```python
from build123d import *

# Parameters (mm, degrees)
SKETCH1_R            = 11
BODY_DEPTH           = 17.5
SKETCH4_W            = 20.5
SKETCH4_H            = 20.5
PROFIL_HOLE_DEPTH    = 20
M4_CLEARANCE_HOLE1_D = 4.5
M5_CLEARANCE_HOLE1_D = 5.5
ELEVATION_START      = 4
SKETCH10_W           = 50
SKETCH10_H           = 50
SKETCH10_R           = 2.25
SKETCH10_R_2         = 11
ELEVATION_DEPTH      = 4
SKETCH11_R           = 3.2
INSERTS_HOLES_DEPTH  = 9.5
SKETCH12_R           = 4.5
M5_VIS_PLACE_DEPTH   = 5
SKETCH13_R           = 3.75
M4_SCREW_PLACE_DEPTH = 4
CHAMFER1_SIZE        = 1


with BuildPart() as part:
    # Sketch1 → Body (new, symmetric)
    with BuildSketch(Plane.XY):
        Polygon((-25, 25), (-15, 45), (15, 45), (25, 25), (25, -25), (-25, -25), align=None)
        Circle(SKETCH1_R, mode=Mode.SUBTRACT)
    extrude(amount=BODY_DEPTH, both=True)

    # Sketch4 → Profil_Hole (cut)
    with BuildSketch(Plane(origin=(0, 45, 0), x_dir=(1, 0, 0), z_dir=(0, 1, 0))):
        Rectangle(SKETCH4_W, SKETCH4_H)
    extrude(amount=-PROFIL_HOLE_DEPTH, mode=Mode.SUBTRACT)

    # M4 Clearance Hole1 (through all)
    with Locations(Plane(origin=(0, 0, -17.5), x_dir=(-1, 0, 0), z_dir=(0, 0, -1))):
        with Locations((0, 0), (-14.25, 14.25), (14.25, -14.25), (14.25, 14.25), (-14.25, -14.25)):
            Hole(M4_CLEARANCE_HOLE1_D / 2)

    # M5 Clearance Hole1 (through all)
    with Locations(Plane(origin=(0, 0, -17.5), x_dir=(-1, 0, 0), z_dir=(0, 0, -1))):
        with Locations((0, 40), (0, 30)):
            Hole(M5_CLEARANCE_HOLE1_D / 2)

    # Sketch10 → Elevation (add)
    with BuildSketch(Plane.XY.offset(17.5).offset(ELEVATION_START)):
        Rectangle(SKETCH10_W, SKETCH10_H)
        with Locations(Location((-14.25, -14.25, 0), (0, 0, 180))):
            Circle(SKETCH10_R, mode=Mode.SUBTRACT)
        with Locations(Location((14.25, -14.25, 0), (0, 0, 180))):
            Circle(SKETCH10_R, mode=Mode.SUBTRACT)
        with Locations(Location((14.25, 14.25, 0), (0, 0, 180))):
            Circle(SKETCH10_R, mode=Mode.SUBTRACT)
        Circle(SKETCH10_R_2, mode=Mode.SUBTRACT)
        with Locations(Location((-14.25, 14.25, 0), (0, 0, 180))):
            Circle(SKETCH10_R, mode=Mode.SUBTRACT)
    extrude(amount=-ELEVATION_DEPTH)

    # Sketch11 → Inserts_Holes (cut)
    with BuildSketch(Plane(origin=(0, 0, -17.5), x_dir=(-1, 0, 0), z_dir=(0, 0, -1))):
        with Locations((-18, 0)):
            Circle(SKETCH11_R)
        with Locations(Location((18, 0, 0), (0, 0, 180))):
            Circle(SKETCH11_R)
    extrude(amount=-INSERTS_HOLES_DEPTH, mode=Mode.SUBTRACT)

    # Sketch12 → M5_Vis_Place (cut)
    with BuildSketch(Plane(origin=(0, 0, -17.5), x_dir=(-1, 0, 0), z_dir=(0, 0, -1))):
        with Locations((0, 40)):
            Circle(SKETCH12_R)
        with Locations((0, 30)):
            Circle(SKETCH12_R)
    m5_vis_place = extrude(amount=-M5_VIS_PLACE_DEPTH, mode=Mode.SUBTRACT)

    # Mirror1: M5_Vis_Place across plane
    add(m5_vis_place.mirror(Plane.XY), mode=Mode.SUBTRACT)

    # Sketch13 → M4_Screw_Place (cut)
    with BuildSketch(Plane(origin=(0, 0, -17.5), x_dir=(-1, 0, 0), z_dir=(0, 0, -1))):
        with Locations((-14.25, 14.25)):
            Circle(SKETCH13_R)
        with Locations((14.25, 14.25)):
            Circle(SKETCH13_R)
        with Locations((14.25, -14.25)):
            Circle(SKETCH13_R)
        with Locations((-14.25, -14.25)):
            Circle(SKETCH13_R)
    extrude(amount=-M4_SCREW_PLACE_DEPTH, mode=Mode.SUBTRACT)

    # Chamfer1
    chamfer1_edges = [part.edges().sort_by_distance(p)[0] for p in [
        (0, 25, 21.5),
    ]]
    chamfer(chamfer1_edges, length=CHAMFER1_SIZE)


solid = part.part
```
Can you work these out from the model? Positions are in its coordinate system, mm. A direction names the side the tool comes from. Give positions to 0.01 mm unless a question says otherwise; leave off trailing zeros. Write each loop counter-clockwise with the first axis right and the second up, starting at its lowest first coordinate (ties: lowest second). Pieces come first, ordered by that corner, then holes. Notation, with made-up numbers: (-1, 34.5) - (46, 34.5) arc R8 ccw to (46, 44.5) - close; hole circle Ø3 at (81, -1). An arc over 180 degrees is marked (long way). Write item = value, one per line. Start each with the question number.
1. Imagine slicing it at C-C (y = 30). Please give me the cut outline in (x, z), and give its area (3 significant figures).
2. Thinking about a two-plate mould opening in X: for faces 1 (the face through (25, 0, 2)), 2 (the face through (0, 35, -10.25)), 3 (the face through (0, 35, 17.5)), 4 (the face through (11.8, 14.3, -13.5)), which applies, released by +X, released by -X, zero draft, split by the parting line, or undercut?
3. Imagine slicing it at D-D (x = -7). Please give me the cut outline in (y, z).
4. For pin 1 (4 mm diameter, centred on x = -14.25, y = -14.25, fed in from +Z); pin 2 (5 mm diameter, centred on x = -17, z = -2, fed in from +Y); pin 3 (6 mm diameter, centred on x = 14.25, y = -14.25, fed in from -Z); pin 4 (10 mm diameter, centred on x = 4, z = -3, fed in from +Y), each with a flat end and sliding along its axis, tell me the tip position at first contact or that it passes through.
5. On a 3-axis mill with a long thin cutter (end or side, diameter ignored), from which of +Z, -Z, +X, -X, +Y, -Y can I reach the whole of each face in a straight line? I mean faces 5 (the face through (0.98, 35.61, 15.04)), 6 (the face through (-0.358, 32.727, -11.359)), 7 (the face through (0, 25, 0)), 8 (the face through (-3, 40, -12.5)). Say none if no direction works.
6. Imagine slicing it at A-A (y = 14.25). Please give me the cut outline in (x, z), and give its area (4 significant figures).
7. Imagine slicing it at B-B (z = 18.5). Please give me the cut outline in (x, y).
8. Please list where these lines run through material, in increasing order: line 1 (Y direction, x = 14.25, z = 19.2); line 2 (Y direction, x = 0, z = -16.1); line 3 (Y direction, x = 0, z = 12).
Worked answers:
q1.outline = (-22.5, -17.5) - (-4.5, -17.5) - (-4.5, -12.5) - (-2.75, -12.5) - (-2.75, -10.25) - (-10.25, -10.25) - (-10.25, 10.25) - (-2.75, 10.25) - (-2.75, 12.5) - (-4.5, 12.5) - (-4.5, 17.5) - (-22.5, 17.5) - close; (2.75, -12.5) - (4.5, -12.5) - (4.5, -17.5) - (22.5, -17.5) - (22.5, 17.5) - (4.5, 17.5) - (4.5, 12.5) - (2.75, 12.5) - (2.75, 10.25) - (10.25, 10.25) - (10.25, -10.25) - (2.75, -10.25) - close
q1.area = 1,040 mm2
q2.face_1 = released by +X
q2.face_2 = undercut
q2.face_3 = zero draft
q2.face_4 = undercut
q3.outline = (-25, -17.5) - (-8.49, -17.5) - (-8.49, 21.5) - (-25, 21.5) - close; (8.49, -17.5) - (45, -17.5) - (45, -10.25) - (25, -10.25) - (25, 10.25) - (45, 10.25) - (45, 17.5) - (25, 17.5) - (25, 20.5) - (24, 21.5) - (8.49, 21.5) - close
q4.pin_1 = through
q4.pin_2 = 45
q4.pin_3 = -13.5
q4.pin_4 = 25
q5.face_5 = +Z
q5.face_6 = +Z, -Z
q5.face_7 = +Y
q5.face_8 = -Z
q6.outline = (-25, -17.5) - (-18, -17.5) - (-18, -13.5) - (-16.5, -13.5) - (-16.5, 21.5) - (-25, 21.5) - close; (-12, -13.5) - (-10.5, -13.5) - (-10.5, -17.5) - (10.5, -17.5) - (10.5, -13.5) - (12, -13.5) - (12, 21.5) - (-12, 21.5) - close; (16.5, -13.5) - (18, -13.5) - (18, -17.5) - (25, -17.5) - (25, 21.5) - (16.5, 21.5) - close
q6.area = 1,575 mm2
q7.outline = (-25, -25) - (25, -25) - (25, 25) - (-25, 25) - close; hole circle Ø4.5 at (-14.25, -14.25); hole circle Ø4.5 at (-14.25, 14.25); hole circle Ø22 at (0, 0); hole circle Ø4.5 at (14.25, -14.25); hole circle Ø4.5 at (14.25, 14.25)
q8.line_1 = -25 to -16.5, -12 to 12, 16.5 to 25
q8.line_2 = -25 to -11, 11 to 25.5, 34.5 to 35.5, 44.5 to 45
q8.line_3 = -25 to -11, 11 to 27.25, 32.75 to 37.25, 42.75 to 45
